Geometry: final body of the model. Coordinates: model frame, mm. A direction names the side the tool comes from. Round coordinates to 2 decimals unless told otherwise and drop trailing zeros. Order: outer loops, then holes, each group sorted by start corner. A loop starts at its lowest first (then second) coordinate and runs counter-clockwise, first axis right, second up. Notation, with made-up numbers: (70.25, 67) - (127.25, 67) arc R21 ccw to (127.25, 94) - close; hole circle Ø6 at (-13.5, 55). An arc over 180 degrees is marked (long way). Put each result on its own line as item: value. Start each with the question number.
(1) Material intervals for L1, parallel to Z at x = -10, y = 19.5; L2, parallel to Y at x = -15.75, z = -5; L3, parallel to Y at x = -16.75, z = 28, sorted ascending. Write a range as [from, to].
(2) Section D-D (z = 35). Output: boundary loops of the cut face in (x, y), and give its area (3 significant figures).
(3) Pull-direction query (Y, two-part tool) for faces 4 (the face through (-15.084, -0.166, 40.953)), 5 (the face through (-24.154, -0.531, 21.778)), 6 (the face through (-18, 0, 48.61)); classes: released by +Y, released by -Y, zero draft, split by the parting line, or undercut.
(4) Access query for faces 1 (the face through (-15, -15, 30)), 2 (the face through (-8, 17, -6)), 3 (the face through (-11, -9, -10)). Directions: +Z, -Z, +X, -X, +Y, -Y. A direction counts if a zero-diameter tool reaches every point of the face in a straight line with its end or side. Return the directions, or none.
(5) Pin query (flat end, axial travel): P1, Ø3.5, axis at x = -21, y = -2, coming from the -Z side; P2, Ø1.5, axis at x = -20, z = 9.5, coming from the +Y side; P3, Ø3, axis at y = 4.5, z = 30, coming from the +X side. Return the tip coordinate at first contact, or that it passes through.
(6) Section C-C (y = 0). Output: boundary loops of the cut face in (x, z), and give its area (3 significant figures).
(7) Section A-A (z = -15). Output: boundary loops of the cut face in (x, y).
(8) Section B-B (x = -2.25). Output: boundary loops of the cut face in (y, z).
from build123d import *

# Parameters (mm, degrees)
REVOLUTION001_ANGLE = 90
PAD_DEPTH           = 20
SKETCH003_W         = 14
SKETCH003_H         = 12.160038
POCKET_DEPTH        = 24.1610380001
SKETCH004_R         = 2
POCKET001_DEPTH     = 54.611
SKETCH007_W         = 25
SKETCH007_H         = 18
POCKET002_DEPTH     = 20


with BuildPart() as part:
    # Sketch001 → Revolution001 (revolve, symmetric)
    with BuildSketch(Plane.XZ) as revolution001_sk:
        with BuildLine():
            Line((-13.8660806584, 42.1124829734), (-15.7024671828, 47.8455523549))
            ThreePointArc((-15.7024671828, 47.8455523549), (-16.1016197671, 48.3985683965), (-16.750038, 48.61))
            Line((-16.750038, 48.61), (-23.140038, 48.61))
            ThreePointArc((-23.140038, 48.61), (-23.8612869168, 48.3112489168), (-24.160038, 47.59))
            Line((-24.160038, 47.59), (-24.160038, 0))
            Line((-24.160038, 0), (-19.160038, 0))
            Line((-19.160038, 0), (-19.160038, 39.34))
            ThreePointArc((-18.5753612917, 40.0873655582), (-18.9965027288, 39.8144476079), (-19.160038, 39.34))
            Line((-18.5753612917, 40.0873655582), (-14.4211735138, 41.1174742446))
            ThreePointArc((-14.4211735138, 41.1174742446), (-13.9277334111, 41.4945364128), (-13.8660806584, 42.1124829734))
        make_face()
    revolve(axis=Axis((0, 0, 0), (0, 0, 1)), revolution_arc=REVOLUTION001_ANGLE / 2)
    revolve(revolution001_sk.sketch, axis=Axis((0, 0, 0), (0, 0, -1)), revolution_arc=REVOLUTION001_ANGLE / 2)

    # Sketch002 (on Face8 of Revolution001) → Pad (new body)
    with BuildSketch(Plane(origin=(0, 0, 0), x_dir=(1, 0, 0), z_dir=(0, 0, -1))):
        with BuildLine():
            ThreePointArc((0, 24.160038), (-24.160038, 0), (0, -24.160038))
            Line((0, -9), (0, -24.160038))
            ThreePointArc((0, 9), (-9, 0), (0, -9))
            Line((0, 24.160038), (0, 9))
        make_face()
    extrude(amount=PAD_DEPTH)

    # Sketch003 (on Face13 of Pad) → Pocket (cut, through all)
    with BuildSketch(Plane(origin=(0, 0, 0), x_dir=(0, 0, 1), z_dir=(1, 0, 0))):
        with Locations((-13, 18.080019)):
            Rectangle(SKETCH003_W, SKETCH003_H)
        with Locations((-13, -18.080019)):
            Rectangle(SKETCH003_W, SKETCH003_H)
    extrude(amount=-POCKET_DEPTH, mode=Mode.SUBTRACT)

    # Sketch004 (on Face20 of Pocket) → Pocket001 (cut, through all)
    with BuildSketch(Plane(origin=(0, 0, -6), x_dir=(1, 0, 0), z_dir=(0, 0, -1))):
        with Locations((-10, -5)):
            Circle(SKETCH004_R)
    extrude(amount=-POCKET001_DEPTH, mode=Mode.SUBTRACT)

    # Sketch007 (on Face18 of Pocket001) → Pocket002 (cut)
    with BuildSketch(Plane(origin=(0, 0, -20), x_dir=(1, 0, 0), z_dir=(0, 0, -1))):
        with Locations((-12.5, 0)):
            Rectangle(SKETCH007_W, SKETCH007_H)
    extrude(amount=-POCKET002_DEPTH, mode=Mode.SUBTRACT)


solid = part.part
Checks:
1. L1: z = [-6, 0]
1. L2: y = [-18.32, -9], [9, 18.32]
1. L3: y = [-16.75, -9.3], [9.3, 16.75]
2. outline: (-17.08, -17.08) - (-13.55, -13.55) arc R19.16 cw to (-13.55, 13.55) - (-17.08, 17.08) arc R24.16 ccw to start
2. area: 170 mm²
3. face 4: undercut
3. face 5: split by the parting line
3. face 6: zero draft
4. face 1: +Z, +X, -Y
4. face 2: -Z, +X, -X, +Y
4. face 3: -Z, +X, -X
5. P1: stops at z = 0
5. P2: stops at y = 14.6
5. P3: stops at x = -18.2
6. outline: (-24.16, 0) - (-19.16, 0) - (-19.16, 39.34) arc R0.77 cw to (-18.58, 40.09) - (-14.42, 41.12) arc R0.78 ccw to (-13.87, 42.11) - (-15.7, 47.85) arc R1.1 ccw to (-16.75, 48.61) - (-23.14, 48.61) arc R1.02 ccw to (-24.16, 47.59) - close
6. area: 278 mm²
7. outline: (-22.42, -9) arc R24.16 ccw to (-20.97, -12) - (0, -12) - (0, -9) - close; (-22.42, 9) - (0, 9) - (0, 12) - (-20.97, 12) arc R24.16 ccw to start
8. outline: (-24.06, -6) - (-12, -6) - (-12, -20) - (-9, -20) - (-9, 0) - (-24.06, 0) - close; (9, -20) - (12, -20) - (12, -6) - (24.06, -6) - (24.06, 0) - (9, 0) - close
